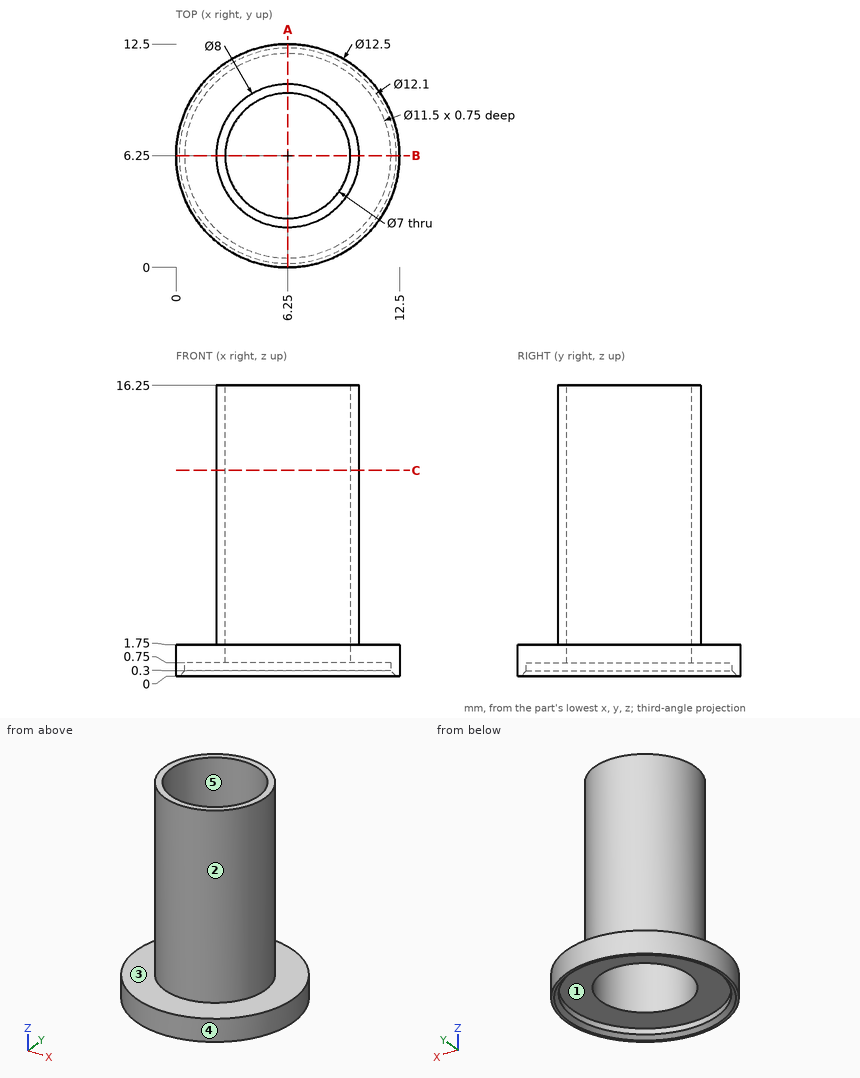
Drawing for the job (mm, zero at the part's lowest x, y, z). A direction names the side the tool comes from. Give positions to 0.01 mm unless a question says otherwise; leave off trailing zeros. Write each loop counter-clockwise with the first axis right and the second up, starting at its lowest first coordinate (ties: lowest second). Pieces come first, ordered by that corner, then holes. Notation, with made-up numbers: (15, -21.75) -> (28, -21.75) arc R28 cw to (28, -2.75) -> close; hole circle Ø10 at (76.25, 29.25). An arc over 180 degrees is marked (long way). Put each result on its own line as item: value. Start each with the question number.
Item 1: Cut at C-C (z = 11.5). List the corners of the cut face in (x, y), then the cut area to 3 significant figures.
Item 2: Cut at A-A (x = 6.25). List the corners of the cut face in (y, z).
Item 3: Pull direction Y, two halves, no side cores. Call the marked faces 3, 4 and 5: pulls with the +Y half, pulls with the -Y half, needs draft (parallel to the pull), parting line crosses it, or undercut.
Item 4: Pin check, flat tips, straight feed: pin 1 Ø3 at (x, y) = (6.5, 3.5) entering from -Z; pin 2 Ø1.5 at (y, z) = (4, 5) entering from +X; pin 3 Ø4 at (x, z) = (6, 6.5) entering from -Y; pin 4 Ø6 at (x, y) = (5, 4.5) entering from +Z. Stop position of each tip, or through.
Item 5: Wall check: L1, parallel to X at y = 6.25, z = 0.6; L2, parallel to Y at x = 6.25, z = 7.25. Give the ranges that are in metal, low to high. Write a range as [from, to].
Item 6: Which spindle directions (+Z, -Z, +X, -X, +Y, -Y) get a long thin tool onto all of the face, cutting with end or side? Do the marked faces 1 and 2. Say none if no direction does.
Answer list:
1. outline: circle Ø8 at (6.25, 6.25); hole circle Ø7 at (6.25, 6.25)
1. area: 11.8 mm2
2. outline: (0, 0) -> (0.2, 0) -> (0.5, 0.3) -> (0.5, 0.75) -> (2.75, 0.75) -> (2.75, 16.25) -> (2.25, 16.25) -> (2.25, 1.75) -> (0, 1.75) -> close; (9.75, 0.75) -> (12, 0.75) -> (12, 0.3) -> (12.3, 0) -> (12.5, 0) -> (12.5, 1.75) -> (10.25, 1.75) -> (10.25, 16.25) -> (9.75, 16.25) -> close
3. face 3: needs draft
3. face 4: parting line crosses it
3. face 5: undercut
4. pin 1: stops at z = 0.75
4. pin 2: stops at x = 9.96
4. pin 3: stops at y = 2.25
4. pin 4: stops at z = 16.25
5. L1: x = [0, 0.5], [12, 12.5]
5. L2: y = [2.25, 2.75], [9.75, 10.25]
6. face 1: -Z
6. face 2: +Z
